Input: part model. Units: mm. Frame: model coordinates. A direction names the side the tool comes from. Coordinates: 2 decimals unless noted, no trailing zeros. Write each loop counter-clockwise with the first axis right and the second up, starting at its lowest first coordinate (ties: lowest second). Pieces come first, ordered by that corner, then holes. Notation, with made-up numbers: (12.25, 60) - (43.25, 60) arc R31 cw to (43.25, 85) - close; hole circle Ø7 at (88, -29.5). An arc over 180 degrees is marked (long way). Use a Markdown table: item, result. Add a question column.
Q1. Pin query (flat end, axial travel): P1, Ø1.5, axis at y = -9, z = 1, coming from the +X side; P2, Ø1.5, axis at x = 1, z = 1.5, coming from the -Y side; P3, Ø0.9, axis at y = -12, z = 1.5, coming from the -X side. Return the tip coordinate at first contact, or that it passes through.
Q2. Set-up query: faces 5 (the face through (0, -47, 2)), 6 (the face through (-7.5, -38, 1)), 7 (the face through (-6.184, 10.919, 1.479)). Return all of +Z, -Z, +X, -X, +Y, -Y with unobstructed straight access to the full face (end or side cutting, diameter ignored); none if empty.
Q3. Mould query, pull axis Y, two halves, no side actions, for faces 1 (the face through (-0.1, -108.5, 1.5)), 2 (the face through (7.5, -5, 1)), 3 (the face through (-3.248, 10.221, 1.479)), 4 (the face through (8.1, -11.2, 1.5)). Classes: released by +Y, released by -Y, zero draft, split by the parting line, or undercut.
Q4. Section query C-C (y = -16). Return the cut outline in (x, z), then the cut area to 3 significant figures.
Q5. Material intervals for probe 1 along X at (y, z) = (-9, 0.25); probe 2 along Y at (x, z) = (-11, 0.45); probe 3 along X at (y, z) = (-57, 2.45), sorted ascending. Write a range as from..to.
Q6. Section query D-D (z = 1.25). Give the number of separate pieces and of enclosed holes in the cut face, then the cut area to 3 significant figures.
Q7. Section query B-B (y = -56). Return the cut outline in (x, z), then the cut area to 3 significant figures.
Q8. Section query A-A (y = -90). Return the cut outline in (x, z), then the cut area to 3 significant figures.
from build123d import *

# Parameters (mm, degrees)
SKETCH_1_R          = 1.575
SKETCH_1_R_2        = 14.5
EXTRUDE_1_DEPTH     = 3
CUT_EXTRUDE_START   = -3
CUT_EXTRUDE_1_DEPTH = 3
SKETCH_3_W          = 9
SKETCH_3_H          = 4
EXTRUDE_2_DEPTH     = 3
SKETCH_4_R          = 4
SKETCH_4_R_2        = 1.4
EXTRUDE_3_DEPTH     = 3
FILLET_1_R          = 2
FILLET_2_R          = 10
FILLET_3_R          = 2.5
CUT_EXTRUDE_2_DEPTH = 10


with BuildPart() as part:
    # 草图1 → 凸台-拉伸1 (new body)
    with BuildSketch(Plane.XY):
        with BuildLine():
            ThreePointArc((7.5, 0), (7.485279444, 0.469671844), (7.441175562, 0.9375))
            Line((7.441175562, 0.9375), (4.960783708, 20.625))
            ThreePointArc((4.960783708, 20.625), (0, 25), (-4.960783708, 20.625))
            Line((-4.960783708, 20.625), (-7.441175562, 0.9375))
            ThreePointArc((-7.441175562, 0.9375), (-7.485279444, 0.469671844), (-7.5, 0))
            Line((-7.5, 0), (-7.5, -69.31788212))
            ThreePointArc((-7.5, -69.31788212), (0, -112), (7.5, -69.31788212))
            Line((7.5, -69.31788212), (7.5, 0))
        make_face()
        with Locations((-12.374368671, -102.374368671)):
            Circle(SKETCH_1_R, mode=Mode.SUBTRACT)
        with Locations((-12.374368671, -77.625631329)):
            Circle(SKETCH_1_R, mode=Mode.SUBTRACT)
        with Locations((0, -90)):
            Circle(SKETCH_1_R_2, mode=Mode.SUBTRACT)
        with Locations((12.374368671, -102.374368671)):
            Circle(SKETCH_1_R, mode=Mode.SUBTRACT)
        with Locations((12.374368671, -77.625631329)):
            Circle(SKETCH_1_R, mode=Mode.SUBTRACT)
        Circle(SKETCH_1_R, mode=Mode.SUBTRACT)
        with Locations((0, 20)):
            Circle(SKETCH_1_R, mode=Mode.SUBTRACT)
    extrude(amount=EXTRUDE_1_DEPTH)

    # 草图2 → 切除-拉伸1 (cut)
    with BuildSketch(Plane.XY.offset(3).offset(CUT_EXTRUDE_START)):
        with BuildLine():
            Line((0, -68), (0, -5))
            ThreePointArc((0, -5), (-2.655442773, -4.236581603), (-4.5, -2.179449472))
            Line((-4.5, -2.179449472), (-4.5, -68.465144533))
            ThreePointArc((-4.5, -68.465144533), (-2.261988032, -68.116595097), (0, -68))
        make_face()
        with BuildLine():
            ThreePointArc((4.5, -2.179449472), (2.655442773, -4.236581603), (0, -5))
            Line((0, -5), (0, -68))
            ThreePointArc((0, -68), (2.261988032, -68.116595097), (4.5, -68.465144533))
            Line((4.5, -68.465144533), (4.5, -2.179449472))
        make_face()
        with BuildLine():
            Line((-2.557135445, 15.70336663), (-4.192274153, 2.724855487))
            ThreePointArc((-4.192274153, 2.724855487), (0, 5), (4.192274153, 2.724855487))
            Line((4.192274153, 2.724855487), (2.557135445, 15.70336663))
            ThreePointArc((2.557135445, 15.70336663), (0, 15), (-2.557135445, 15.70336663))
        make_face()
    extrude(amount=CUT_EXTRUDE_1_DEPTH, mode=Mode.SUBTRACT)

    # 草图3 → 凸台-拉伸2 (add)
    with BuildSketch(Plane.XY.offset(3)):
        with Locations((0, -45)):
            Rectangle(SKETCH_3_W, SKETCH_3_H)
        with Locations((0, -25)):
            Rectangle(SKETCH_3_W, SKETCH_3_H)
    extrude(amount=-EXTRUDE_2_DEPTH)

    # 草图4 → 凸台-拉伸3 (add)
    # profile 1 of 4: a face of its own
    with BuildSketch(Plane.XY.offset(3)):
        with Locations((-9, -16)):
            Circle(SKETCH_4_R)
        with Locations((-9, -16)):
            Circle(SKETCH_4_R_2, mode=Mode.SUBTRACT)
    # profile 2 of 4: a face of its own
    with BuildSketch(Plane.XY.offset(3)):
        with Locations((-9, -61.2)):
            Circle(SKETCH_4_R)
        with Locations((-9, -61.2)):
            Circle(SKETCH_4_R_2, mode=Mode.SUBTRACT)
    # profile 3 of 4: a face of its own
    with BuildSketch(Plane.XY.offset(3)):
        with Locations((9, -61.2)):
            Circle(SKETCH_4_R)
        with Locations((9, -61.2)):
            Circle(SKETCH_4_R_2, mode=Mode.SUBTRACT)
    # profile 4 of 4: a face of its own
    with BuildSketch(Plane.XY.offset(3)):
        with Locations((9, -16)):
            Circle(SKETCH_4_R)
        with Locations((9, -16)):
            Circle(SKETCH_4_R_2, mode=Mode.SUBTRACT)
    extrude(amount=-EXTRUDE_3_DEPTH)

    # 圆角1
    fillet_1_edges = [part.edges().sort_by_distance(p)[0] for p in [
        (-4.5, -27, 1.5),
        (-4.5, -23, 1.5),
        (4.5, -23, 1.5),
        (4.5, -27, 1.5),
        (-2.557135445, 15.70336663, 1.5),
        (2.557135445, 15.70336663, 1.5),
        (4.192274153, 2.724855487, 1.5),
        (-4.192274153, 2.724855487, 1.5),
        (4.5, -68.465144533, 1.5),
        (-4.5, -68.465144533, 1.5),
        (-4.5, -2.179449472, 1.5),
        (4.5, -2.179449472, 1.5),
        (-4.5, -47, 1.5),
        (-4.5, -43, 1.5),
        (4.5, -43, 1.5),
        (4.5, -47, 1.5),
    ]]
    fillet(fillet_1_edges, radius=FILLET_1_R)

    # 圆角2
    # the kernel refuses this fillet: 10 mm, written as the material it adds along each edge
    with BuildSketch(Plane(origin=(-7.5, -69.31788212, 0), x_dir=(-0.8959663420766752, -0.44412195832422213, 0), z_dir=(0, 0, 1))) as fillet_2_piece_1:
        with BuildLine():
            CenterArc((6.0520135, -9.936998269), FILLET_2_R, 96.434905118, 46.795533404)
            Line((-1.958481407, -3.951017033), (-2.118691305, -3.831297409))
            ThreePointArc((-2.118691305, -3.831297409), (-1.158433972, -1.886684125), (-0.179193268, 0.088824392))
            Line((-0.179193268, 0.088824392), (0.022414865, 0.198739965))
            ThreePointArc((0.022414865, 0.198739965), (2.46563513, 0.061396191), (4.908855394, 0.198739965))
            Line((4.908855394, 0.198739965), (4.931270259, 0))
        make_face()
    extrude(amount=3)
    with BuildSketch(Plane(origin=(7.5, -69.31788212, 0), x_dir=(0.8959663420766733, -0.44412195832422613, 0), z_dir=(0, 0, 1))) as fillet_2_piece_2:
        with BuildLine():
            CenterArc((6.0520135, 9.936998269), FILLET_2_R, 216.769561479, 46.795533404)
            Line((-1.958481407, 3.951017033), (-2.118691305, 3.831297409))
            ThreePointArc((-2.118691305, 3.831297409), (-1.158433972, 1.886684125), (-0.179193268, -0.088824392))
            Line((-0.179193268, -0.088824392), (0.022414865, -0.198739965))
            ThreePointArc((0.022414865, -0.198739965), (2.46563513, -0.061396191), (4.908855394, -0.198739965))
            Line((4.908855394, -0.198739965), (4.931270259, 0))
        make_face()
    extrude(amount=3)

    # 圆角3
    fillet_3_edges = [part.edges().sort_by_distance(p)[0] for p in [
        (-7.5, -64.908099244, 1.5),
        (-7.5, -57.491900756, 1.5),
        (7.5, -64.908099244, 1.5),
        (7.5, -57.491900756, 1.5),
        (-7.5, -12.291900756, 1.5),
        (-7.5, -19.708099244, 1.5),
        (7.5, -12.291900756, 1.5),
        (7.5, -19.708099244, 1.5),
    ]]
    fillet(fillet_3_edges, radius=FILLET_3_R)

    # 草图5 → 切除-拉伸2 (cut)
    with BuildSketch(Plane.XY.offset(3)):
        with BuildLine():
            ThreePointArc((8.848308271, -73.753232914), (0, -71.5), (-8.848308271, -73.753232914))
            ThreePointArc((-8.848308271, -73.753232914), (-9.248224964, -75.109723474), (-7.891734404, -75.509640167))
            ThreePointArc((-7.891734404, -75.509640167), (1.6e-08, -73.5), (7.891734432, -75.509640182))
            ThreePointArc((7.891734432, -75.509640182), (9.248224971, -75.10972346), (8.848308271, -73.753232914))
        make_face()
        with BuildLine():
            ThreePointArc((16.246767086, -81.151691729), (14.890276526, -80.751775036), (14.490359833, -82.108265596))
            ThreePointArc((14.490359833, -82.108265596), (16.5, -90.000000016), (14.490359818, -97.891734432))
            ThreePointArc((14.490359818, -97.891734432), (14.89027654, -99.248224971), (16.246767086, -98.848308271))
            ThreePointArc((16.246767086, -98.848308271), (18.5, -90), (16.246767086, -81.151691729))
        make_face()
        with BuildLine():
            ThreePointArc((8.848308271, -106.246767086), (9.248224964, -104.890276526), (7.891734404, -104.490359833))
            ThreePointArc((7.891734404, -104.490359833), (-1.6e-08, -106.5), (-7.891734432, -104.490359818))
            ThreePointArc((-7.891734432, -104.490359818), (-9.248224971, -104.89027654), (-8.848308271, -106.246767086))
            ThreePointArc((-8.848308271, -106.246767086), (0, -108.5), (8.848308271, -106.246767086))
        make_face()
        with BuildLine():
            ThreePointArc((-16.246767086, -98.848308271), (-14.890276526, -99.248224964), (-14.490359833, -97.891734404))
            ThreePointArc((-14.490359833, -97.891734404), (-16.5, -89.999999984), (-14.490359818, -82.108265568))
            ThreePointArc((-14.490359818, -82.108265568), (-14.89027654, -80.751775029), (-16.246767086, -81.151691729))
            ThreePointArc((-16.246767086, -81.151691729), (-18.5, -90), (-16.246767086, -98.848308271))
        make_face()
    extrude(amount=-CUT_EXTRUDE_2_DEPTH, mode=Mode.SUBTRACT)


solid = part.part
Values follow:
| question | item | result |
|---|---|---|
| 1 | P1 | x = 7.51 |
| 1 | P2 | y = -112 |
| 1 | P3 | x = -10.84 |
| 2 | face 5 | +Z, -Z |
| 2 | face 6 | +Z, -Z, -X |
| 2 | face 7 | +Z, -Z, -X, +Y |
| 3 | face 1 | undercut |
| 3 | face 2 | zero draft |
| 3 | face 3 | undercut |
| 3 | face 4 | released by +Y |
| 4 | outline | (-13, 0) - (-10.4, 0) - (-10.4, 3) - (-13, 3) - close; (-7.6, 0) - (-4.5, 0) - (-4.5, 3) - (-7.6, 3) - close; (4.5, 0) - (7.6, 0) - (7.6, 3) - (4.5, 3) - close; (10.4, 0) - (13, 0) - (13, 3) - (10.4, 3) - close |
| 4 | area | 34.2 mm2 |
| 5 | probe 1 | -7.5..-4.5, 4.5..7.5 |
| 5 | probe 2 | -109.05..-103.14, -101.61..-99.45, -80.55..-78.39, -76.86..-70.84, -64.66..-57.74, -19.46..-12.54 |
| 5 | probe 3 | -8.86..-4.5, 4.5..8.86 |
| 6 | separate pieces | 1 |
| 6 | enclosed holes | 19 |
| 6 | area | 1,570 mm2 |
| 7 | outline | (-7.82, 0) - (-4.5, 0) - (-4.5, 3) - (-7.82, 3) - close; (4.5, 0) - (7.82, 0) - (7.82, 3) - (4.5, 3) - close |
| 7 | area | 19.9 mm2 |
| 8 | outline | (-22, 0) - (-18.5, 0) - (-18.5, 3) - (-22, 3) - close; (-16.5, 0) - (-14.5, 0) - (-14.5, 3) - (-16.5, 3) - close; (14.5, 0) - (16.5, 0) - (16.5, 3) - (14.5, 3) - close; (18.5, 0) - (22, 0) - (22, 3) - (18.5, 3) - close |
| 8 | area | 33.0 mm2 |
